Design review of the part built by this model. Coordinates are the model's own, in mm. A direction names the side the tool comes from. Round coordinates to 2 decimals unless told otherwise and drop trailing zeros. Order: outer loops, then holes, each group sorted by start corner. A loop starts at its lowest first (then second) coordinate and runs counter-clockwise, first axis right, second up. Notation, with made-up numbers: (15, 66) - (59, 66) arc R23 cw to (59, 102) - close; hole circle Ø9 at (69.5, 83.5). An arc over 180 degrees is marked (long way). Write item = value, one per line.
from build123d import *

# Parameters (mm, degrees)
CYLINDER012_R     = 14.5
CYLINDER012_DEPTH = 1
PAD_DEPTH         = 3.5
CYLINDER011_R     = 2.25
CYLINDER011_DEPTH = 10
ARRAY002_COUNT    = 5
CYLINDER010_R     = 24
CYLINDER010_DEPTH = 5.5


with BuildPart() as cylinder012:
    # Cylinder012 → Cylinder012 (new body)
    with BuildSketch(Plane.XY.offset(20)):
        Circle(CYLINDER012_R)
    extrude(amount=CYLINDER012_DEPTH)


with BuildPart() as obj1:
    # Sketch → Pad (new body)
    with BuildSketch(Plane.XY):
        Polygon((4, 0), (2, 3.464102), (-2, 3.464102), (-4, 0), (-2, -3.464102), (2, -3.464102), align=None)
    extrude(amount=PAD_DEPTH)


with BuildPart() as obj1_1:
    # Body placement: moved
    add(obj1.part.moved(Location((19, 0, 22))))


with BuildPart() as array002:
    # Cylinder011 → Cylinder011 (new body)
    with BuildSketch(Plane(origin=(19, 0, 20), x_dir=(1, 0, 0), z_dir=(0, 0, 1))):
        Circle(CYLINDER011_R)
    extrude(amount=CYLINDER011_DEPTH)

    # Fusion003: union obj1
    add(obj1_1.part)

    # Array002: Array002 ×5 about axis
    array002_axis = Axis((0, 0, 0), (0, 0, 1))


with BuildPart() as array002_1:
    add(array002.part)
    for i in range(1, ARRAY002_COUNT):
        add(array002.part.rotate(array002_axis, i * 360 / ARRAY002_COUNT))


with BuildPart() as cut006:
    # Cylinder010 → Cylinder010 (new body)
    with BuildSketch(Plane.XY.offset(20)):
        Circle(CYLINDER010_R)
    extrude(amount=CYLINDER010_DEPTH)

    # Cut005: cut Array002
    add(array002_1.part, mode=Mode.SUBTRACT)

    # Cut006: cut Cylinder012
    add(cylinder012.part, mode=Mode.SUBTRACT)


solid = cut006.part
Item 1: Take a section at C-C, the plane x = 5.5. State the section outline as (y, z) points, and give its area (3 significant figures).
Data:
outline = (-23.36, 20) - (-20.29, 20) - (-20.29, 22) - (-21.53, 22) - (-21.53, 25.5) - (-23.36, 25.5) - close; (-15.85, 20) - (-13.42, 20) - (-13.42, 21) - (13.42, 21) - (13.42, 20) - (15.85, 20) - (15.85, 22) - (14.45, 22) - (14.45, 25.5) - (-14.45, 25.5) - (-14.45, 22) - (-15.85, 22) - close; (20.29, 20) - (23.36, 20) - (23.36, 25.5) - (21.53, 25.5) - (21.53, 22) - (20.29, 22) - close
area = 163 mm2
Item 2: Take a section at B-B, the plane x = 0. State the section outline as (y, z) points.
Data:
outline = (-24, 20) - (-14.5, 20) - (-14.5, 21) - (14.5, 21) - (14.5, 20) - (24, 20) - (24, 25.5) - (-24, 25.5) - close
Item 3: For line 1 along Y through (x, z) = (5, 20.55); line 2 along X through (y, z) = (13, 20.4); line 3 along Y through (x, z) = (7.5, 22.8), list the stretches that pass through material, from the lowest coordinate up. Write a range as [from, to].
Data:
line_1 = [-23.47, -20.14], [-16, -13.61], [13.61, 16], [20.14, 23.47]
line_2 = [-20.17, -16.68], [-14.07, -6.42], [6.42, 20.17]
line_3 = [-22.8, -21.44], [-14.87, 14.87], [21.44, 22.8]
Item 4: Insertion check: P1, Ø17.5, axis at x = 0, y = 0, coming from the -Z side; P2, Ø2, axis at x = -18.5, z = 23.5, coming from the +Y side; P3, Ø3, axis at x = 18, z = 23.5, coming from the -Y side. Each pin has a flat end and moves straight along its axis. Give the tip position at first contact, or say it passes through.
Data:
P1 = 21
P2 = 16.42
P3 = -17.43
Item 5: Take a section at A-A, the plane z = 24.7. Count the separate pieces of the cut face and the enclosed holes in it, and give its area (3 significant figures).
Data:
separate_pieces = 1
enclosed_holes = 5
area = 1,600 mm2
Item 6: The part is to be moulded in two halves that separate along Y. For faces 1 (the face through (5.178, 21.464, 23.726)), 2 (the face through (0, 0, 25.5)), say which applies: +Y half, -Y half, draft (parallel to the pull), parting line (faces both ways), or undercut.
Data:
face_1 = undercut
face_2 = draft
Item 7: For faces 3 (the face through (6.691, -12.864, 20.493)), 4 (the face through (-11.93, 10.78, 23.73)), 5 (the face through (6.62, 15.95, 20.99)), list the 3-axis set-ups (+Z, -Z, +X, -X, +Y, -Y) from which the entire face can be reached by the end or side of a thin tool; tool diameter is ignored.
Data:
face_3 = -Z
face_4 = +Z
face_5 = +Z, -Z
Item 8: Take a section at D-D, the plane y = -11. State the section outline as (x, z) points, and give its area (3 significant figures).
Data:
outline = (-21.33, 20) - (-17.62, 20) - (-17.62, 22) - (-18.87, 22) - (-18.87, 25.5) - (-21.33, 25.5) - close; (-13.13, 20) - (-9.45, 20) - (-9.45, 21) - (9.45, 21) - (9.45, 20) - (21.33, 20) - (21.33, 25.5) - (-11.91, 25.5) - (-11.91, 22) - (-13.13, 22) - close
area = 182 mm2
